Verification items for this drawing (mm, ordinates from the low corner). Round coordinates to 2 decimals unless told otherwise and drop trailing zeros. Order: outer loops, then holes, each group sorted by start corner. A loop starts at its lowest first (then second) coordinate and runs counter-clockwise, first axis right, second up. Notation, with made-up numbers: (26, -23) - (79, -23) arc R11 ccw to (79, -12) - close; hole circle Ø8 at (68.5, 84). An arc over 180 degrees is marked (long way). Return JSON: item names as keys, results as strings. Group by question number.
Q1. Sectioned sample at D-D, the plane z = 7.75. Record the cut outline in (x, y), then the cut area to 3 significant figures.
Q2. Material ranges on line 1 along Y through (x, z) = (9, 3.5); line 2 along Y through (x, z) = (5, 2.5); line 3 along X through (y, z) = (12.5, 5.75), recorded low to high.
Q3. Gauge pin test, flat ends, axial feed: pin 1 Ø1 at (x, z) = (12.5, 2.5) entering from -Y; pin 2 Ø2.5 at (y, z) = (9, 4) entering from -X; pin 3 Ø1.5 at (y, z) = (15.5, 3) entering from +X. Record the tip position at first contact, or that the pin passes through.
Q4. Sectioned sample at C-C, the plane y = 4.5. Record the cut outline in (x, z).
Q5. Draft check along X on the marked faces 1, 2, 3 and 4. Enter one of: pulls with the +X half, pulls with the -X half, needs draft (parallel to the pull), parting line crosses it, or undercut.
Q6. Sectioned sample at A-A, the plane y = 9. Record the cut outline in (x, z), then the cut area to 3 significant figures.
Q7. Sectioned sample at B-B, the plane x = 11. Record the cut outline in (y, z), then the cut area to 3 significant figures.
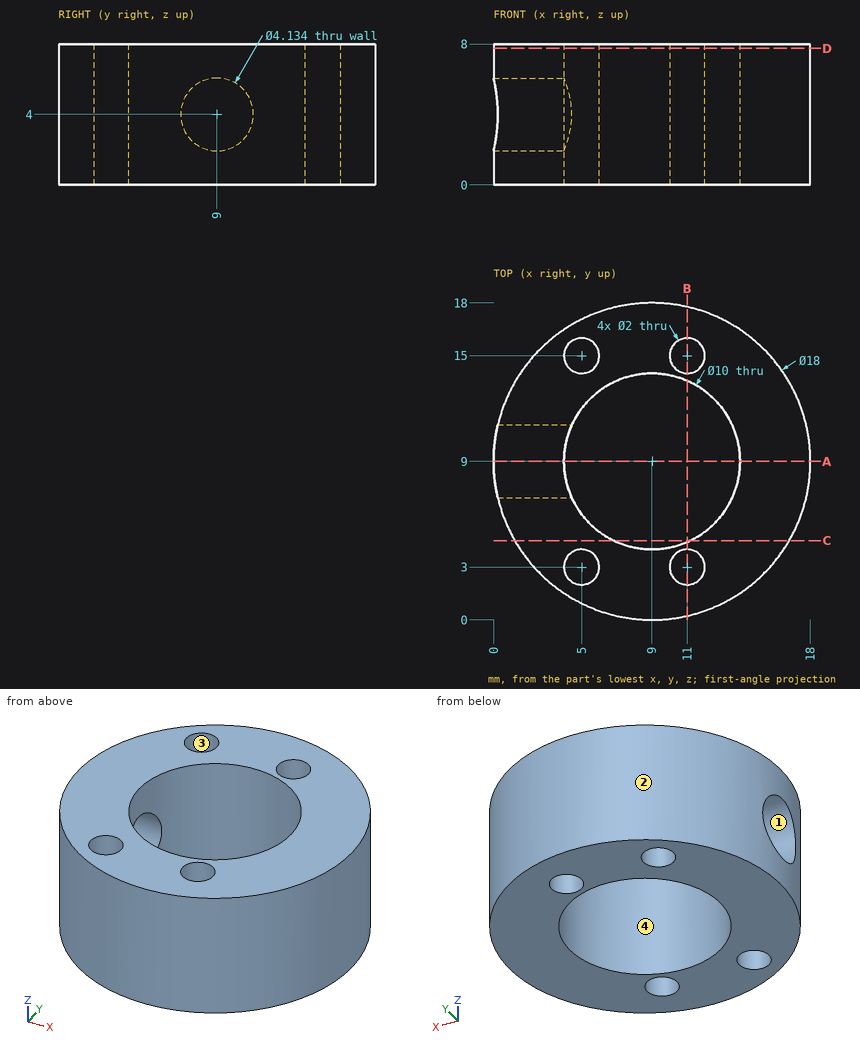
Reply:
{
 "1": {"outline": "circle Ø18 at (9, 9); hole circle Ø2 at (5, 3); hole circle Ø10 at (9, 9); hole circle Ø2 at (5, 15); hole circle Ø2 at (11, 3); hole circle Ø2 at (11, 15)", "area": "163 mm^2"},
 "2": {"line 1": "0 to 4, 14 to 18", "line 2": "0.94 to 2, 4 to 6, 12 to 14, 16 to 17.06", "line 3": "0.71 to 5.43, 12.57 to 17.29"},
 "3": {"pin 1": "y = 0.51", "pin 2": "x = 13.84", "pin 3": "x = 15.92"},
 "4": {"outline": "(1.21, 0) - (6.82, 0) - (6.82, 8) - (1.21, 8) - close; (11.18, 0) - (16.79, 0) - (16.79, 8) - (11.18, 8) - close"},
 "5": {"face 1": "needs draft", "face 2": "parting line crosses it", "face 3": "undercut", "face 4": "undercut"},
 "6": {"outline": "(0, 0) - (4, 0) - (4, 1.93) - (0, 1.93) - close; (0, 6.07) - (4, 6.07) - (4, 8) - (0, 8) - close; (14, 0) - (18, 0) - (18, 8) - (14, 8) - close", "area": "47.5 mm^2"},
 "7": {"outline": "(0.23, 0) - (2, 0) - (2, 8) - (0.23, 8) - close; (4, 0) - (4.42, 0) - (4.42, 8) - (4, 8) - close; (13.58, 0) - (14, 0) - (14, 8) - (13.58, 8) - close; (16, 0) - (17.77, 0) - (17.77, 8) - (16, 8) - close", "area": "35.1 mm^2"}
}
